Autodesk Inventor part; units mm, degrees
ref_plane "YZ Plane" through (0, 0, 0) normal (1, 0, 0) x (0, 1, 0)
ref_plane "XZ Plane" through (0, 0, 0) normal (0, 1, 0) x (-1, 0, 0)
ref_plane "XY Plane" through (0, 0, 0) normal (0, 0, 1) x (1, 0, 0)
sketch "Sketch2" plane through (0, 0, 0) normal (0, 1, 0) x (-1, 0, 0)
  line L0 (11.45, 1.45) -> (0, 1.45)
  line L1 (0, 1.45) -> (0, -10.5)
  line L2 (0, -10.5) -> (11.45, -10.5)
  line L3 (11.45, -10.5) -> (11.45, 1.45)
  line L4 (1.75, 0) -> (1.75, -8.25)
  line L5 (0, 0) -> (1.75, 0) construction
  line L6 (1.75, -8.25) -> (0, -8.25) construction
  line L7 (0, 0) -> (1.75, -0.3086)
  line L8 (0, -8.25) -> (1.75, -7.9414)
  line L9 (0, 0) -> (0, -8.25)
  dimension "d9" = 0
  dimension "d10" = 11.45
  dimension "d11" = 11.95
  dimension "d12" = 10.5
  dimension "d13" = 1.75
  dimension "d14" = 8.25
  dimension "d15" = 10
  dimension "d16" = 10
extrude "Extrusion2" add sketch "Sketch2" along normal blind 1.68 contours L3 L2 L1 L8 L4 L7 L0
sketch "Sketch3" plane through (0, 0, 1.45) normal (1, 0, 0) x (0, 0, -1)
  line L0 (11.95, 0) -> (0, 0)
  line L1 (11.3835, 0) -> (0.3835, 0)
  line L2 (0.3835, 0) -> (0.3835, 1.15)
  line L3 (0.3835, 1.15) -> (11.3835, 1.15)
  line L4 (11.3835, 1.15) -> (11.3835, 0)
  point P0 (1.45, 0)
  dimension "d19" = 11
  dimension "d20" = 1.15
extrude "Extrusion3" cut sketch "Sketch3" against normal blind 9.15
sketch "Sketch4" plane through (-1.75, 1.68, -0.3086) normal (1, 0, 0) x (0, 0, -1)
  line L0 (-1.3751, -1.68) -> (-1.3751, -0.53)
  line L1 (9.6249, -1.68) -> (-1.3751, -1.68)
  line L2 (-1.3751, -1.48) -> (9.6249, -1.48)
  line L3 (9.6249, -1.48) -> (9.6249, -1.68)
  line L4 (9.6249, -1.68) -> (-1.3751, -1.68)
  line L5 (-1.3751, -1.68) -> (-1.3751, -1.48)
  line L6 (0, -0.53) -> (7.6329, -0.53)
  line L7 (3.8164, -0.53) -> (5.5042, -0.53)
  point P0 (-0.3086, -1.68)
  dimension "d23" = 0.95
extrude "Extrusion4" add sketch "Sketch4" against normal up to next
sketch "Sketch5" plane through (0, 0, 0) normal (0, 0, 1) x (1, 0, 0)
  line L0 (-2, 0.15) -> (-0.4808, 0.15)
  line L1 (-0.4808, 0.15) -> (-0.4467, 0.1)
  line L2 (-0.4467, 0.1) -> (0, 0.1)
  line L3 (0, 0.1) -> (0, -0.05)
  line L4 (0, -0.05) -> (-0.5, -0.05)
  line L5 (-0.5, -0.05) -> (-0.5341, 0)
  line L6 (-0.5341, 0) -> (-2, 0)
  line L7 (-2, 0) -> (-2, 0.15)
  point P0 (0, 0)
  dimension "d26" = 0
  dimension "d27" = 0.5
  dimension "d28" = 2
  dimension "d29" = 0.05
  dimension "d30" = 0.15
  dimension "d32" = 0.15
  dimension "d33" = 0.2
extrude "Extrusion5" add sketch "Sketch5" along normal mid plane 0.3
pattern_linear "Rectangular Pattern1" count 8 spacing 1.1 along (0, 0, -1) of "Extrusion5"
properties part number "uSDCard"
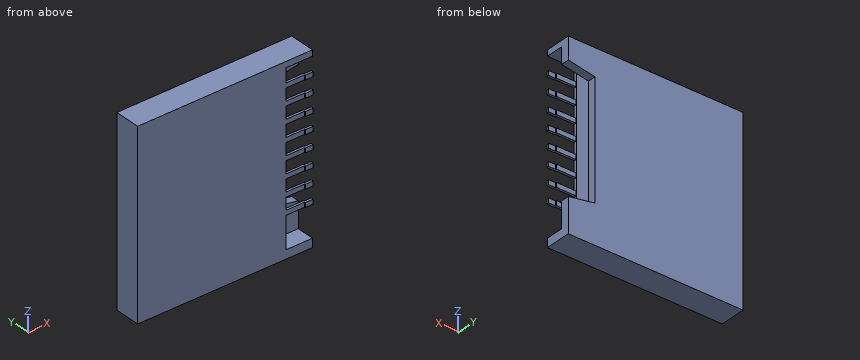
The model under review builds one solid part; all positions refer to its coordinate system, in mm. Give positions to 0.01 mm unless a question says otherwise; leave off trailing zeros. Order: outer loops, then holes, each group sorted by start corner. A loop starts at its lowest first (then second) coordinate and runs counter-clockwise, first axis right, second up. Notation, with made-up numbers: M -39.75,25.5 L -29.75,25.5 A25 cw -29.75,63.5 Z; hole C 26.5,-14.5 d3. An arc over 180 degrees is marked long. Use one line per item in the form item = value. Start each with the question number.
Item 1: We need section D-D on y = 1.5. Give the boundary of the cut face in (x, z), plus the area to 3 significant figures.
Item 2: To check wall thickness, follow line 1 along Z through (x, y) = (-5, 0.25); line 2 along Y through (x, z) = (-7.75, -6.25); line 3 along Y through (x, z) = (-1.25, -9.5). State the ranges of each line that lie inside material, in increasing order. Write a range as from..to.
Item 3: Insertion check: pin 1 Ø5.5 at (x, z) = (-3.5, -7) entering from -Y; pin 2 Ø1 at (y, z) = (1, -4.5) entering from +X; pin 3 Ø6 at (x, z) = (-1.5, -3.5) entering from +Y. Each pin has a flat end and moves straight along its axis. Give the tip position at first contact, or say it passes through.
Item 4: We need section B-B on z = -5.5. Give the boundary of the cut face in (x, y), plus the area to 3 significant figures.
Item 5: We need section C-C on y = 0.5. Give the boundary of the cut face in (x, z).
Item 6: We need section A-A on x = -3. Give the boundary of the cut face in (y, z).
Completed:
q1.outline = M -11.45,-10.5 L 0,-10.5 L 0,-8.25 L -1.75,-7.94 L -1.75,-0.31 L 0,0 L 0,1.45 L -11.45,1.45 Z
q1.area = 123 mm²
q2.line_1 = -10.5..-9.93, 1.07..1.45
q2.line_2 = 0..0.2, 1.15..1.68
q2.line_3 = 1.15..1.68
q3.pin_1 = 0
q3.pin_2 = -1.75
q3.pin_3 = 1.68
q4.outline = M -11.45,0 L -0.53,0 L -0.5,-0.05 L 0,-0.05 L 0,0.1 L -0.45,0.1 L -0.48,0.15 L -1.75,0.15 L -1.75,0.2 L -9.15,0.2 L -9.15,1.15 L -1.75,1.15 L -1.75,1.68 L -11.45,1.68 Z
q4.area = 9.53 mm²
q5.outline = M -11.45,-10.5 L 0,-10.5 L 0,-9.93 L -9.15,-9.93 L -9.15,1.07 L 0,1.07 L 0,1.45 L -11.45,1.45 Z
q6.outline = M 0,-10.5 L 1.68,-10.5 L 1.68,1.45 L 0,1.45 Z; hole M 0.2,-9.93 L 1.15,-9.93 L 1.15,1.07 L 0.2,1.07 Z
